Could you check a few things on this model? Use its own coordinates, in mm. A direction names the side the tool comes from. Give positions to 0.01 mm unless a question says otherwise; leave off trailing zeros. Loops run counter-clockwise (first coordinate to the right, second up) from the corner with the lowest first, then second, coordinate; pieces in that order, holes last. Notation, with made-up numbers: (17.5, -19) - (42.5, -19) arc R26 ccw to (42.5, 13) - close; hole circle Ø11 at (47, 58.5). An arc over 180 degrees is marked (long way). Write each question's results on one line, items separated by ' | '. Start each with the question number.
```python
from build123d import *

# Parameters (mm, degrees)
BOSS_EXTRUDE1_DEPTH = 12.7
SKETCH2_R           = 1.7018
CUT_EXTRUDE1_DEPTH  = 56.896


with BuildPart() as part:
    # Sketch1 → Boss-Extrude1 (new body)
    with BuildSketch(Plane.XZ.offset(6.35)):
        with BuildLine():
            ThreePointArc((3.900741532, 6.293125734), (2.850773823, 5.595435975), (2.180140266, 4.527983952))
            ThreePointArc((2.180140266, 4.527983952), (1.71882223, 4.722425266), (1.240447645, 4.870004095))
            ThreePointArc((1.240447645, 4.870004095), (1.41285747, 6.118794727), (1.057001873, 7.328162323))
            ThreePointArc((1.057001873, 7.328162323), (0.645301119, 7.375825545), (0.231578393, 7.400377521))
            ThreePointArc((0.231578393, 7.400377521), (-0.328875436, 6.271176611), (-0.375935122, 5.011419263))
            ThreePointArc((-0.375935122, 5.011419263), (-0.872668917, 4.949151363), (-1.360742875, 4.837771086))
            ThreePointArc((-1.360742875, 4.837771086), (-1.835826903, 6.005460409), (-2.748690687, 6.874875672))
            ThreePointArc((-2.748690687, 6.874875672), (-3.12906561, 6.710302855), (-3.499635989, 6.524704127))
            ThreePointArc((-3.499635989, 6.524704127), (-3.420402788, 5.266560539), (-2.831278997, 4.15204883))
            ThreePointArc((-2.831278997, 4.15204883), (-3.230329132, 3.849756349), (-3.597323441, 3.509261221))
            ThreePointArc((-3.597323441, 3.509261221), (-4.592602939, 4.282967824), (-5.817873798, 4.579471636))
            ThreePointArc((-5.817873798, 4.579471636), (-6.065001736, 4.246759935), (-6.293125734, 3.900741532))
            ThreePointArc((-6.293125734, 3.900741532), (-5.595435975, 2.850773823), (-4.527983952, 2.180140266))
            ThreePointArc((-4.527983952, 2.180140266), (-4.722425266, 1.71882223), (-4.870004095, 1.240447645))
            ThreePointArc((-4.870004095, 1.240447645), (-6.118794727, 1.41285747), (-7.328162323, 1.057001873))
            ThreePointArc((-7.328162323, 1.057001873), (-7.375825545, 0.645301119), (-7.400377521, 0.231578393))
            ThreePointArc((-7.400377521, 0.231578393), (-6.271176611, -0.328875436), (-5.011419263, -0.375935122))
            ThreePointArc((-5.011419263, -0.375935122), (-4.949151363, -0.872668917), (-4.837771086, -1.360742875))
            ThreePointArc((-4.837771086, -1.360742875), (-6.005460409, -1.835826903), (-6.874875672, -2.748690687))
            ThreePointArc((-6.874875672, -2.748690687), (-6.710302855, -3.12906561), (-6.524704127, -3.499635989))
            ThreePointArc((-6.524704127, -3.499635989), (-5.266560539, -3.420402788), (-4.15204883, -2.831278997))
            ThreePointArc((-4.15204883, -2.831278997), (-3.849756349, -3.230329132), (-3.509261221, -3.597323441))
            ThreePointArc((-3.509261221, -3.597323441), (-4.282967824, -4.592602939), (-4.579471636, -5.817873798))
            ThreePointArc((-4.579471636, -5.817873798), (-4.246759935, -6.065001736), (-3.900741532, -6.293125734))
            ThreePointArc((-3.900741532, -6.293125734), (-2.850773823, -5.595435975), (-2.180140266, -4.527983952))
            ThreePointArc((-2.180140266, -4.527983952), (-1.71882223, -4.722425266), (-1.240447645, -4.870004095))
            ThreePointArc((-1.240447645, -4.870004095), (-1.41285747, -6.118794727), (-1.057001873, -7.328162323))
            ThreePointArc((-1.057001873, -7.328162323), (-0.645301119, -7.375825545), (-0.231578393, -7.400377521))
            ThreePointArc((-0.231578393, -7.400377521), (0.328875436, -6.271176611), (0.375935122, -5.011419263))
            ThreePointArc((0.375935122, -5.011419263), (0.872668917, -4.949151363), (1.360742875, -4.837771086))
            ThreePointArc((1.360742875, -4.837771086), (1.835826903, -6.005460409), (2.748690687, -6.874875672))
            ThreePointArc((2.748690687, -6.874875672), (3.12906561, -6.710302855), (3.499635989, -6.524704127))
            ThreePointArc((3.499635989, -6.524704127), (3.420402788, -5.266560539), (2.831278997, -4.15204883))
            ThreePointArc((2.831278997, -4.15204883), (3.230329132, -3.849756349), (3.597323441, -3.509261221))
            ThreePointArc((3.597323441, -3.509261221), (4.592602939, -4.282967824), (5.817873798, -4.579471636))
            ThreePointArc((5.817873798, -4.579471636), (6.065001736, -4.246759935), (6.293125734, -3.900741532))
            ThreePointArc((6.293125734, -3.900741532), (5.595435975, -2.850773823), (4.527983952, -2.180140266))
            ThreePointArc((4.527983952, -2.180140266), (4.722425266, -1.71882223), (4.870004095, -1.240447645))
            ThreePointArc((4.870004095, -1.240447645), (6.118794727, -1.41285747), (7.328162323, -1.057001873))
            ThreePointArc((7.328162323, -1.057001873), (7.375825545, -0.645301119), (7.400377521, -0.231578393))
            ThreePointArc((7.400377521, -0.231578393), (6.271176611, 0.328875436), (5.011419263, 0.375935122))
            ThreePointArc((5.011419263, 0.375935122), (4.949151363, 0.872668917), (4.837771086, 1.360742875))
            ThreePointArc((4.837771086, 1.360742875), (6.005460409, 1.835826903), (6.874875672, 2.748690687))
            ThreePointArc((6.874875672, 2.748690687), (6.710302855, 3.12906561), (6.524704127, 3.499635989))
            ThreePointArc((6.524704127, 3.499635989), (5.266560539, 3.420402788), (4.15204883, 2.831278997))
            ThreePointArc((4.15204883, 2.831278997), (3.849756349, 3.230329132), (3.509261221, 3.597323441))
            ThreePointArc((3.509261221, 3.597323441), (4.282967824, 4.592602939), (4.579471636, 5.817873798))
            ThreePointArc((4.579471636, 5.817873798), (4.246759935, 6.065001736), (3.900741532, 6.293125734))
        make_face()
        with BuildLine():
            Line((1.331822463, 1.588907621), (1.794942153, -1.037574657))
            ThreePointArc((1.794942153, -1.037574657), (1.752865603, -1.227369709), (1.588907621, -1.331822463))
            Line((1.588907621, -1.331822463), (-1.037574657, -1.794942153))
            ThreePointArc((-1.037574657, -1.794942153), (-1.227369709, -1.752865603), (-1.331822463, -1.588907621))
            Line((-1.331822463, -1.588907621), (-1.794942153, 1.037574657))
            ThreePointArc((-1.794942153, 1.037574657), (-1.752865603, 1.227369709), (-1.588907621, 1.331822463))
            Line((-1.588907621, 1.331822463), (1.037574657, 1.794942153))
            ThreePointArc((1.037574657, 1.794942153), (1.227369709, 1.752865603), (1.331822463, 1.588907621))
        make_face(mode=Mode.SUBTRACT)
    extrude(amount=-BOSS_EXTRUDE1_DEPTH)

    # Sketch2 → Cut-Extrude1 (cut)
    with BuildSketch(Plane(origin=(0, 6.35, 0), x_dir=(1, 0, 0), z_dir=(0, 1, 0))):
        Circle(SKETCH2_R)
    extrude(amount=-CUT_EXTRUDE1_DEPTH, mode=Mode.SUBTRACT)


solid = part.part
```
Q1. I need wall thicknesses on L1, parallel to X at y = 1.75, z = 5.5; L2, parallel to Z at x = 5.5, y = -3. Which ranges of each line are inside material? Lowest first, please. Write a range as from..to.
Q2. I'm going to push flat-ended pins straight in: pin 1 Ø1.5 at (y, z) = (4, -3.5) entering from +X; pin 2 Ø4 at (y, z) = (4, 2) entering from -X; pin 3 Ø4 at (x, y) = (3.5, -0.5) entering from -Z; pin 4 Ø5 at (y, z) = (-2, -3) entering from -X. Where does each tip first touch, or does it pass through?
Q3. Which directions (+Z, -Z, +X, -X, +Y, -Y) give clear straight access to the entire face, cutting with the end or side of a thin tool? Please do faces 4 (the face through (-0.651, -0.089, -7.375)), 5 (the face through (1.674, 0.089, 0.304)), 6 (the face through (-1.826, -0.089, 5.991)).
Q4. I want a section at B-B, the plane x = -2.5. List the corners of the cut face in (y, z) for me.
Q5. I want a section at A-A, the plane z = 3.25. List the corners of the cut face in (x, y) for me, then the cut area to 3 significant figures.
Q6. If we mould it in two halves opening along X, with no side actions, what happens to faces 1 (the face through (-7.375, -0.089, 0.651)), 2 (the face through (-6.101, -0.089, 1.414)), 3 (the face through (7.375, -0.089, -0.651))? For each: +X half, -X half, draft (parallel to the pull), parting line (faces both ways), or undercut.
Conclusion:
1) L1: -3.48..-1.56, -0.42..1.39, 2.76..4.55 | L2: -4.55..-2.76, -1.39..0.42, 1.56..3.48
2) pin 1: x = 6.29 | pin 2: x = -7.4 | pin 3: z = -6.87 | pin 4: x = -6.87
3) face 4: -Z, -X, +Y, -Y | face 5: +Y, -Y | face 6: +Z, +Y, -Y
4) outline: (-6.35, -5.16) - (6.35, -5.16) - (6.35, 6.7) - (-6.35, 6.7) - close
5) outline: (-5.94, -6.35) - (3.83, -6.35) - (3.83, 6.35) - (-5.94, 6.35) - close; (4.81, -6.35) - (6.65, -6.35) - (6.65, 6.35) - (4.81, 6.35) - close | area: 148 mm^2
6) face 1: -X half | face 2: undercut | face 3: +X half
